Here's how the part is built. I have some questions about the finished solid (model axes, mm). A direction names the side the tool comes from. Give positions to 0.01 mm unless a question says otherwise; leave off trailing zeros. Order: outer loops, then holes, each group sorted by start corner. A loop starts at its lowest first (then second) coordinate and runs counter-clockwise, first axis right, second up. Notation, with made-up numbers: M 37.25,4 L 42.25,4 A25 cw 42.25,34 Z; hole C -13,83.25 d5. An arc over 180 degrees is marked long. Use one line per item in the form item = value.
from build123d import *

# Parameters (mm, degrees)
SKETCH_3_R          = 10
EXTRUDE_1_DEPTH     = 7
SKETCH_4_R          = 2.5
CUT_EXTRUDE_1_DEPTH = 18


with BuildPart() as part:
    # Эскиз2 → Повернуть1 (revolve)
    with BuildSketch(Plane(origin=(0, 0, 0), x_dir=(0, 0, -1), z_dir=(1, 0, 0))):
        Polygon((0, 0), (0, 21), (1.5, 21), (1.5, 19), (8.5, 19), (8.5, 21), (10, 21), (10, 0), align=None)
    revolve(axis=Axis((0, 0, -10), (0, 0, 1)))

    # Эскиз3 → Бобышка-Вытянуть1 (add)
    with BuildSketch(Plane(origin=(0, 0, -10), x_dir=(-1, 0, 0), z_dir=(0, 0, -1))):
        Circle(SKETCH_3_R)
    extrude(amount=EXTRUDE_1_DEPTH)

    # Эскиз4 → Вырез-Вытянуть1 (cut, through all)
    with BuildSketch(Plane(origin=(0, 0, -17), x_dir=(-1, 0, 0), z_dir=(0, 0, -1))):
        Circle(SKETCH_4_R)
    extrude(amount=-CUT_EXTRUDE_1_DEPTH, mode=Mode.SUBTRACT)


solid = part.part
Q1. I'm going to push flat-ended pins straight in: pin 1 Ø2 at (x, z) = (-12, -11.5) entering from -Y; pin 2 Ø1 at (y, z) = (-5.5, -12) entering from +X; pin 3 Ø1.5 at (x, z) = (-5.5, -2.5) entering from +Y; pin 4 Ø8 at (x, z) = (-11.5, -14.5) entering from -Y. Where does each tip first touch, or does it pass through?
Found:
pin_1 = through
pin_2 = 8.66
pin_3 = 18.4
pin_4 = -6.61
Q2. I want a section at C-C on z = -13.75. Write out the boundary of the cut face in (x, y), then the cut area to 3 significant figures.
Found:
outline = C 0,0 d20; hole C 0,0 d5
area = 295 mm²
Q3. I want a section at D-D on y = -9. Write out the boundary of the cut face in (x, z).
Found:
outline = M -18.97,-10 L -4.36,-10 L -4.36,-17 L 4.36,-17 L 4.36,-10 L 18.97,-10 L 18.97,-8.5 L 16.73,-8.5 L 16.73,-1.5 L 18.97,-1.5 L 18.97,0 L -18.97,0 L -18.97,-1.5 L -16.73,-1.5 L -16.73,-8.5 L -18.97,-8.5 Z
Q4. I need wall thicknesses on L1, parallel to Y at x = 0, z = -8.75; L2, parallel to Y at x = 0, z = -5.25; L3, parallel to Z at x = 10, y = -6. Which ranges of each line are inside material? Lowest first, please.
Found:
L1 = -21 to -2.5, 2.5 to 21
L2 = -19 to -2.5, 2.5 to 19
L3 = -10 to 0
Q5. On a 3-axis mill with a long thin cutter (end or side, diameter ignored), from which of +Z, -Z, +X, -X, +Y, -Y can I reach the whole of each face in a straight line? I mean faces 1 (the face through (11, -16, -1.5)), 2 (the face through (-2, -2, -17)), 3 (the face through (2.17, -9.76, -13.45)). Say none if no direction works.
Found:
face_1 = none
face_2 = -Z, +X, -X, +Y, -Y
face_3 = -Z
Q6. I want a section at A-A on x = 0. Write out the boundary of the cut face in (y, z).
Found:
outline = M -21,-10 L -10,-10 L -10,-17 L -2.5,-17 L -2.5,0 L -21,0 L -21,-1.5 L -19,-1.5 L -19,-8.5 L -21,-8.5 Z; M 2.5,-17 L 10,-17 L 10,-10 L 21,-10 L 21,-8.5 L 19,-8.5 L 19,-1.5 L 21,-1.5 L 21,0 L 2.5,0 Z
Q7. Thinking about a two-plate mould opening in Z: for faces 4 (the face through (16.856, 8.767, -5.049)), 5 (the face through (-5, 9, -10)), 6 (the face through (0, -4, 0)), which applies, +Z half, -Z half, draft (parallel to the pull), parting line (faces both ways), or undercut?
Found:
face_4 = undercut
face_5 = -Z half
face_6 = +Z half
